For this review, take the finished solid that the model builds, in its own axes (mm). Face numbers are marked on the shaded views. Coordinates: 2 decimals unless noted, no trailing zeros. Write each loop counter-clockwise with the first axis right and the second up, starting at its lowest first coordinate (ties: lowest second). Pieces come first, ordered by that corner, then holes. Notation, with made-up numbers: M 72.5,-33.75 L 103.5,-33.75 A31 ccw 103.5,-2.75 Z; hole C 49.25,-26 d7. An arc over 180 degrees is marked long. Return JSON: item names as keys, results as strings.
Autodesk Inventor part; units mm, degrees
ref_plane "YZ Plane" through (0, 0, 0) normal (1, 0, 0) x (0, 1, 0)
ref_plane "XZ Plane" through (0, 0, 0) normal (0, 1, 0) x (-1, 0, 0)
ref_plane "XY Plane" through (0, 0, 0) normal (0, 0, 1) x (1, 0, 0)
sketch "Sketch1" plane through (0, 0, 0) normal (0, 1, 0) x (-1, 0, 0)
  line L0 (-44.45, -19.05) -> (44.45, -19.05)
  line L1 (44.45, -19.05) -> (44.45, 19.05)
  line L2 (44.45, 19.05) -> (-44.45, 19.05)
  line L3 (-44.45, 19.05) -> (-44.45, -19.05)
  line L4 (-44.45, -19.05) -> (44.45, 19.05) construction
  line L5 (44.45, -19.05) -> (-44.45, 19.05) construction
  circle A0 centre (22.225, 0) radius 3.9688
  circle A1 centre (-22.225, 0) radius 3.9688
  circle A2 centre (22.225, 0) radius 12.7
  circle A3 centre (-22.225, 0) radius 12.7
  point P0 (0, 0)
  point P1 (0, 0)
  point P2 (0, 0)
  dimension "d3" = 38.1
  dimension "d4" = 88.9
  dimension "d20" = 7.9375
  dimension "d21" = 25.4
  dimension "d22" = 22.225
  dimension "d23" = 22.225
extrude "Extrusion5" add sketch "Sketch1" along normal blind 25.4 contours L3 L2 L1 L0 | A2 | A3
sketch "Sketch8" plane through (0, 0, 0) normal (0, 0, 1) x (1, 0, 0)
  line L0 (44.45, 25.4) -> (-44.45, 25.4)
  circle A0 centre (-27.9591, 24.13) radius 1.7653
  line L1 (-26.1938, 25.4) -> (-18.2563, 25.4)
  line L2 (-18.2563, 0) -> (-26.1938, 0)
  line L3 (-26.1938, 0) -> (-26.1938, 25.4)
  line L4 (-18.2563, 0) -> (-18.2563, 25.4)
  line L5 (-22.225, 25.4) -> (-22.225, 0) construction
  line L6 (-44.45, 25.4) -> (-44.45, 27.8765) construction
  line L7 (-27.9591, 22.3647) -> (-22.225, 22.3647)
  line L8 (-26.7329, 25.4) -> (-22.225, 25.4) construction
  line L9 (-22.225, 22.3647) -> (-22.225, 25.4)
  line L10 (-22.225, 25.4) -> (-26.7329, 25.4)
  point P0 (0, 0)
  dimension "d34" = 3.5306
  dimension "d35" = 1.27
revolve "Revolution1" cut sketch "Sketch8" angle 360 about axis through (-22.225, 25.4, 0) along (0, -1, 0) contours L9 L7 L3 L0 | L3 A0 L0 | A0 L0 | L0 A0 | L3 L7 A0
sketch "Sketch9" plane through (0, 25.4, 0) normal (0, 1, 0) x (1, 0, 0)
  circle A0 centre (-22.225, 0) radius 6.9602
  circle A1 centre (22.225, 0) radius 3.9687
  line L0 (44.45, 19.05) -> (-44.45, 19.05)
  line L1 (-44.45, 19.05) -> (-44.45, -19.05)
  line L2 (-44.45, -19.05) -> (44.45, -19.05)
  line L3 (44.45, -19.05) -> (44.45, 19.05)
  circle A2 centre (-22.225, 0) radius 4.8006
  point P0 (0, 0)
  dimension "d37" = 9.6012
properties part number "AirPressureAndValve"
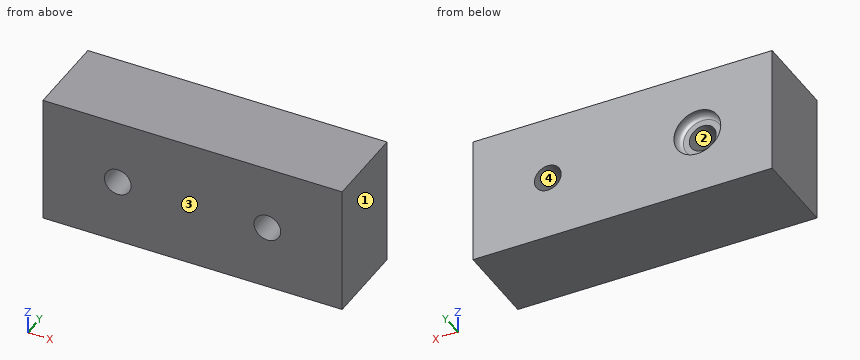
1. Clearance check with flat-ended pins moving along their axes: pin 1 Ø9 at (x, z) = (-22.225, 0) entering from +Y; pin 2 Ø9 at (x, z) = (22.225, 0) entering from +Y; pin 3 Ø4 at (x, z) = (-27, 1) entering from +Y. State where each tip first meets the part, or that it passes through.
Checks:
{"pin 1": "y = 22.36", "pin 2": "y = 25.4", "pin 3": "y = 22.79"}
2. We need section B-B (z = 0). State the section outline as (x, y) points, plus the area to 3 significant figures.
Checks:
{"outline": "M -44.45,0 L -26.19,0 L -26.19,22.36 L -27.96,22.36 A1.77 cw -29.19,25.4 L -44.45,25.4 Z; M -18.26,0 L 18.26,0 L 18.26,25.4 L -15.26,25.4 A1.77 cw -16.49,22.36 L -18.26,22.36 Z; M 26.19,0 L 44.45,0 L 44.45,25.4 L 26.19,25.4 Z", "area": "1,840 mm2"}
3. We need section C-C (x = 25). State the section outline as (y, z) points, plus the area to 3 significant figures.
Checks:
{"outline": "M 0,-19.05 L 25.4,-19.05 L 25.4,-2.84 L 0,-2.84 Z; M 0,2.84 L 25.4,2.84 L 25.4,19.05 L 0,19.05 Z", "area": "824 mm2"}
4. We need section A-A (y = 4.25). State the section outline as (x, z) points (3 decimals).
Checks:
{"outline": "M -44.45,-19.05 L 44.45,-19.05 L 44.45,19.05 L -44.45,19.05 Z; hole C -22.225,0 d7.938; hole C 22.225,0 d7.938"}
5. Draft analysis for pull direction X (two halves, no side actions). For the marked faces 1, 2, 3 and 4, state which applies: +X half, -X half, draft (parallel to the pull), parting line (faces both ways), or undercut.
Checks:
{"face 1": "+X half", "face 2": "undercut", "face 3": "draft", "face 4": "undercut"}
6. Wall thickness on L1, parallel to Z at x = 22.5, y = 10.75; L2, parallel to Z at x = -19, y = 9.5: over which ranges is each line inside the solid? List them lowest first. Write a range as from..to.
Checks:
{"L1": "-19.05..-3.96, 3.96..19.05", "L2": "-19.05..-2.31, 2.31..19.05"}
